Study the drawing (mm; zero at the part's minimum x, y, z) and answer. A direction names the side the tool comes from. Give positions to 0.01 mm unless a question says otherwise; leave off trailing zeros. Write each loop counter-clockwise with the first axis right and the second up, starting at its lowest first coordinate (ties: lowest second). Pieces come first, ordered by that corner, then holes. Notation, with made-up numbers: (52, -36.5) -> (106, -36.5) arc R18 ccw to (106, -10.5) -> close; hole circle Ø8 at (10, 30.5). An arc over 180 degrees is marked (long way). Use CSV: the item, a comma, the result in double quotes. Start each with the question number.
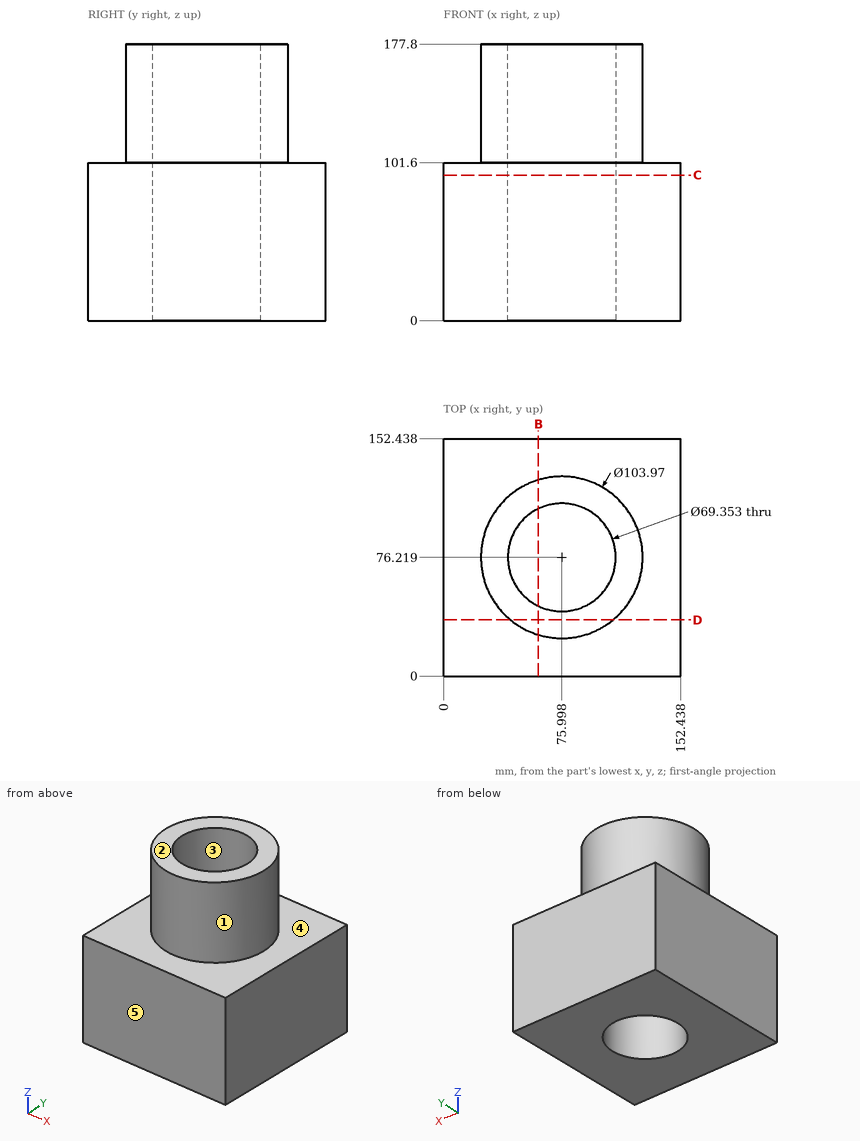
Q1. Straight lines are drawn through the part: L1, parallel to Z at x = 20.5, y = 118.5; L2, parallel to X at y = 50.5, z = 81 (1 decimal); L3, parallel to X at y = 89.5, z = 36.5 (1 decimal). For each, find the intervals that lie inside material, in ascending order.
Q2. Section C-C on z = 93.5 is taken. Give the vertices of the cut face in (x, y) (1 decimal), then the cut area to 3 significant figures.
Q3. The mould has two halves that part along Y. Classify the marked faces 1, 2 and 3: +Y half, -Y half, draft (parallel to the pull), parting line (faces both ways), or undercut.
Q4. Flat-ended cylindrical pins translate along their axes: pin 1 Ø6 at (x, z) = (107, 110.5) entering from +Y; pin 2 Ø4 at (y, z) = (119.5, 141.5) entering from -X; pin 3 Ø5 at (y, z) = (32, 152.5) entering from -X; pin 4 Ø2 at (y, z) = (130.5, 106.5) entering from -X. Find the tip coordinate at first contact, or state that the pin passes through.
Q5. Section D-D on y = 36 is taken. Give the vertices of the cut face in (x, z) (1 decimal), then the cut area to 3 significant figures.
Q6. Section B-B on x = 61 is taken. Give the vertices of the cut face in (y, z) (1 decimal).
Q7. For the marked faces 4 and 5, determine the directions among +Z, -Z, +X, -X, +Y, -Y from which every point of the face is accessible in a straight line to the end or side of a thin tool.
Output:
1,L1,"0 to 101.6"
1,L2,"0 to 52.7, 99.3 to 152.4"
1,L3,"0 to 44, 108 to 152.4"
2,outline,"(0, 0) -> (152.4, 0) -> (152.4, 152.4) -> (0, 152.4) -> close; hole circle Ø69.4 at (76, 76.2)"
2,area,"19,500 mm²"
3,face 1,"parting line"
3,face 2,"draft"
3,face 3,"undercut"
4,pin 1,"y = 120.02"
4,pin 2,"x = 44.4"
4,pin 3,"x = 44.98"
4,pin 4,"through"
5,outline,"(0, 0) -> (152.4, 0) -> (152.4, 101.6) -> (108.9, 101.6) -> (108.9, 177.8) -> (43.1, 177.8) -> (43.1, 101.6) -> (0, 101.6) -> close"
5,area,"20,500 mm²"
6,outline,"(0, 0) -> (45, 0) -> (45, 177.8) -> (26.4, 177.8) -> (26.4, 101.6) -> (0, 101.6) -> close; (107.5, 0) -> (152.4, 0) -> (152.4, 101.6) -> (126, 101.6) -> (126, 177.8) -> (107.5, 177.8) -> close"
7,face 4,"+Z"
7,face 5,"+Z, -Z, +X, -X, -Y"
